from build123d import *
from build123d import SkipClean  # not in build123d's __all__

# Parameters (mm, degrees)
F1_DEPTH = 40
F3_DEPTH = 1.001
F4_DEPTH = 2
F5_DEPTH = 0.5
F6_R     = 0.49999


# Not quite as in the source:
# - a fillet or chamfer is up to 0.001 mm smaller than in the source, because OpenCascade refuses the exact size


with BuildPart() as f1:
    # F0 (on Top) → F1 (new body)
    with BuildSketch(Plane.XY):
        with BuildLine():
            Line((11, 0), (10, 0))
            ThreePointArc((10, 0), (2.4380397486, -9.6982453147), (-8.8111924369, -4.7289415137))
            Line((-8.8111924369, -4.7289415137), (-9.6923116806, -5.2018356651))
            ThreePointArc((-9.6923116806, -5.2018356651), (2.6818437234, -10.6680698462), (11, 0))
        make_face()
        with BuildLine():
            Line((10, 4.582575695), (10, 0))
            Line((10, 0), (11, 0))
            ThreePointArc((11, 0), (10.7470926301, 2.3452078799), (10, 4.582575695))
        make_face()
        with BuildLine():
            Line((10, 16.417424305), (10, 4.582575695))
            ThreePointArc((10, 4.582575695), (10.7470926301, 2.3452078799), (11, 0))
            Line((11, 0), (11, 21))
            ThreePointArc((11, 21), (10.7470926301, 18.6547921201), (10, 16.417424305))
        make_face()
        with BuildLine():
            ThreePointArc((0, 11), (1.6583123952, 10.8742815855), (3.2787192622, 10.5))
            ThreePointArc((3.2787192622, 10.5), (7.2687738933, 12.743794692), (10, 16.417424305))
            Line((10, 16.417424305), (10, 21))
            ThreePointArc((10, 21), (7.0710678119, 13.9289321881), (0, 11))
        make_face()
        with BuildLine():
            ThreePointArc((-3.2787192622, 10.5), (-1.6583124171, 10.1257184179), (-4.44e-08, 10))
            ThreePointArc((-4.44e-08, 10), (1.6583123732, 10.1257184112), (3.2787192622, 10.5))
            ThreePointArc((3.2787192622, 10.5), (1.6583123952, 10.8742815855), (0, 11))
            ThreePointArc((0, 11), (-1.6583123952, 10.8742815855), (-3.2787192622, 10.5))
        make_face()
        with BuildLine():
            ThreePointArc((-9.6923116806, 15.7981643349), (-7.0056796429, 12.5194072884), (-3.2787192622, 10.5))
            ThreePointArc((-3.2787192622, 10.5), (-1.6583123952, 10.8742815855), (0, 11))
            ThreePointArc((0, 11), (-5.1337405886, 12.4183505333), (-8.8111924369, 16.2710584863))
            Line((-8.8111924369, 16.2710584863), (-9.6923116806, 15.7981643349))
        make_face()
        with BuildLine():
            Line((10, 21), (10, 16.417424305))
            ThreePointArc((10, 16.417424305), (10.7470926301, 18.6547921201), (11, 21))
            ThreePointArc((11, 21), (10.7470926301, 23.3452078799), (10, 25.582575695))
            Line((10, 25.582575695), (10, 21))
        make_face()
        with BuildLine():
            ThreePointArc((10, 25.582575695), (10.7470926301, 23.3452078799), (11, 21))
            Line((11, 21), (11, 42))
            ThreePointArc((11, 42), (10.7470926301, 39.6547921201), (10, 37.417424305))
            Line((10, 37.417424305), (10, 25.582575695))
        make_face()
        with BuildLine():
            ThreePointArc((5.81e-08, 32), (1.6583124239, 31.8742815811), (3.2787192622, 31.5))
            ThreePointArc((3.2787192622, 31.5), (7.2687738933, 33.743794692), (10, 37.417424305))
            Line((10, 37.417424305), (10, 42))
            ThreePointArc((10, 42), (7.0710678324, 34.9289322087), (5.81e-08, 32))
        make_face()
        with BuildLine():
            ThreePointArc((5.81e-08, 32), (-1.6583123665, 31.8742815898), (-3.2787192622, 31.5))
            ThreePointArc((-3.2787192622, 31.5), (-1.658312379, 31.1257184121), (3.28e-08, 31))
            ThreePointArc((3.28e-08, 31), (1.6583124114, 31.125718417), (3.2787192622, 31.5))
            ThreePointArc((3.2787192622, 31.5), (1.6583124239, 31.8742815811), (5.81e-08, 32))
        make_face()
        with BuildLine():
            ThreePointArc((-9.6923116806, 36.7981643349), (-7.0056796429, 33.5194072884), (-3.2787192622, 31.5))
            ThreePointArc((-3.2787192622, 31.5), (-1.6583123665, 31.8742815898), (5.81e-08, 32))
            ThreePointArc((5.81e-08, 32), (-5.1337405637, 33.4183505184), (-8.8111924369, 37.2710584863))
            Line((-8.8111924369, 37.2710584863), (-9.6923116806, 36.7981643349))
        make_face()
        with BuildLine():
            ThreePointArc((10, 37.417424305), (10.7470926301, 39.6547921201), (11, 42))
            ThreePointArc((11, 42), (10.7470926301, 44.3452078799), (10, 46.582575695))
            Line((10, 46.582575695), (10, 42))
            Line((10, 42), (10, 37.417424305))
        make_face()
        with BuildLine():
            ThreePointArc((10, 46.582575695), (10.7470926301, 44.3452078799), (11, 42))
            Line((11, 42), (11, 63))
            ThreePointArc((11, 63), (10.7470926301, 60.6547921201), (10, 58.417424305))
            Line((10, 58.417424305), (10, 46.582575695))
        make_face()
        with BuildLine():
            ThreePointArc((10, 58.417424305), (10.7470926301, 60.6547921201), (11, 63))
            ThreePointArc((11, 63), (10.8000300748, 65.0879057409), (10.2073908395, 67.0998990536))
            Line((10.2073908395, 67.0998990536), (10, 67.0998990536))
            Line((10, 67.0998990536), (10, 63))
            Line((10, 63), (10, 58.417424305))
        make_face()
        with BuildLine():
            ThreePointArc((0, 53), (1.6583123952, 52.8742815855), (3.2787192622, 52.5))
            ThreePointArc((3.2787192622, 52.5), (7.2687738933, 54.743794692), (10, 58.417424305))
            Line((10, 58.417424305), (10, 63))
            ThreePointArc((10, 63), (7.0710678119, 55.9289321881), (0, 53))
        make_face()
        with BuildLine():
            ThreePointArc((-5.66e-08, 52), (1.6583123672, 52.1257184103), (3.2787192622, 52.5))
            ThreePointArc((3.2787192622, 52.5), (1.6583123952, 52.8742815855), (0, 53))
            ThreePointArc((0, 53), (-1.6583123952, 52.8742815855), (-3.2787192622, 52.5))
            ThreePointArc((-3.2787192622, 52.5), (-1.6583124232, 52.1257184188), (-5.66e-08, 52))
        make_face()
        with BuildLine():
            ThreePointArc((-9.6923116806, 57.7981643349), (-7.0056796429, 54.5194072884), (-3.2787192622, 52.5))
            ThreePointArc((-3.2787192622, 52.5), (-1.6583123952, 52.8742815855), (0, 53))
            ThreePointArc((0, 53), (-5.1337405886, 54.4183505333), (-8.8111924369, 58.2710584863))
            Line((-8.8111924369, 58.2710584863), (-9.6923116806, 57.7981643349))
        make_face()
        with BuildLine():
            ThreePointArc((10, 67.582575695), (10.1065773297, 67.3424756395), (10.2073908395, 67.0998990536))
            Line((10.2073908395, 67.0998990536), (11, 67.0998990536))
            Line((11, 67.0998990536), (11, 89.784912765))
            Line((11, 89.784912765), (10, 89.784912765))
            Line((10, 89.784912765), (10, 67.582575695))
        make_face()
        with BuildLine():
            ThreePointArc((10.2073908395, 67.0998990536), (10.8000300748, 65.0879057409), (11, 63))
            Line((11, 63), (11, 67.0998990536))
            Line((11, 67.0998990536), (10.2073908395, 67.0998990536))
        make_face()
        with BuildLine():
            Line((10, 67.0998990536), (10.2073908395, 67.0998990536))
            ThreePointArc((10.2073908395, 67.0998990536), (10.1065773297, 67.3424756395), (10, 67.582575695))
            Line((10, 67.582575695), (10, 67.0998990536))
        make_face()
    extrude(amount=F1_DEPTH)

    # F2 (on face) → F3 (cut, through all)
    with BuildSketch(Plane(origin=(10, 0, 0), x_dir=(0, -1, 0), z_dir=(-1, 0, 0))):
        Polygon((-81.784912765, 10.7769520171), (-81.784912765, 0), (-63, 0), align=None)
        with BuildLine():
            Line((-89.784912765, 0), (-81.784912765, 0))
            Line((-81.784912765, 0), (-81.784912765, 10.7769520171))
            Line((-81.784912765, 10.7769520171), (-85.7659138368, 13.0608624119))
            ThreePointArc((-85.7659138368, 13.0608624119), (-88.7076293046, 15.9905117892), (-89.784912765, 20))
            Line((-89.784912765, 20), (-89.784912765, 0))
        make_face()
        with BuildLine():
            Line((-89.784912765, 40), (-89.784912765, 20))
            ThreePointArc((-89.784912765, 20), (-88.7076292465, 24.0094883112), (-85.7659136356, 26.9391377035))
            Line((-85.7659136356, 26.9391377035), (-81.784912765, 29.2230479829))
            Line((-81.784912765, 29.2230479829), (-81.784912765, 40))
            Line((-81.784912765, 40), (-89.784912765, 40))
        make_face()
        Polygon((-81.784912765, 29.2230479829), (-63, 40), (-81.784912765, 40), align=None)
    extrude(amount=-F3_DEPTH, mode=Mode.SUBTRACT)

    # F2 (on face) → F4 (join)
    with BuildSketch(Plane(origin=(10, 0, 0), x_dir=(0, -1, 0), z_dir=(-1, 0, 0))):
        with BuildLine():
            ThreePointArc((-85.7659138368, 13.0608624119), (-83.8448762714, 12.2697638877), (-81.784912765, 12))
            Line((-81.784912765, 12), (-81.784912765, 12.5))
            ThreePointArc((-81.784912765, 12.5), (-89.284912765, 20), (-81.784912765, 27.5))
            Line((-81.784912765, 27.5), (-81.784912765, 28))
            ThreePointArc((-81.784912765, 28), (-83.8448761593, 27.7302361422), (-85.7659136356, 26.9391377035))
            ThreePointArc((-85.7659136356, 26.9391377035), (-88.7076292465, 24.0094883112), (-89.784912765, 20))
            ThreePointArc((-89.784912765, 20), (-88.7076293046, 15.9905117892), (-85.7659138368, 13.0608624119))
        make_face()
        with BuildLine():
            Line((-81.784912765, 12.5), (-81.784912765, 12))
            ThreePointArc((-81.784912765, 12), (-76.1280585155, 14.3431457505), (-73.784912765, 20))
            ThreePointArc((-73.784912765, 20), (-76.1280585155, 25.6568542495), (-81.784912765, 28))
            Line((-81.784912765, 28), (-81.784912765, 27.5))
            ThreePointArc((-81.784912765, 27.5), (-76.4816119061, 25.3033008589), (-74.284912765, 20))
            ThreePointArc((-74.284912765, 20), (-76.4816119061, 14.6966991411), (-81.784912765, 12.5))
        make_face()
    with SkipClean():  # cleaning this boolean's faces spoils the solid; the shape is the same uncleaned
        extrude(amount=F4_DEPTH)

    # F2 (on face) → F5 (cut)
    with BuildSketch(Plane(origin=(10, 0, 0), x_dir=(0, -1, 0), z_dir=(-1, 0, 0))):
        with BuildLine():
            Line((-81.784912765, 27.5), (-81.784912765, 12.5))
            ThreePointArc((-81.784912765, 12.5), (-76.4816119061, 14.6966991411), (-74.284912765, 20))
            ThreePointArc((-74.284912765, 20), (-76.4816119061, 25.3033008589), (-81.784912765, 27.5))
        make_face()
        with BuildLine():
            ThreePointArc((-81.784912765, 27.5), (-89.284912765, 20), (-81.784912765, 12.5))
            Line((-81.784912765, 12.5), (-81.784912765, 27.5))
        make_face()
    with SkipClean():  # cleaning this boolean's faces spoils the solid; the shape is the same uncleaned
        extrude(amount=-F5_DEPTH, mode=Mode.SUBTRACT)

    # F6 (radius 0.5 in the source; OpenCascade refuses exactly that, so slightly less here)
    f6_edges = [f1.edges().sort_by_distance(p)[0] for p in [
        (-8.811192, 58.271058, 20),
        (-9.692312, 57.798164, 20),
        (-8.811192, 37.271058, 20),
        (-9.692312, 36.798164, 20),
        (-8.811192, 16.271058, 20),
        (-9.692312, 15.798164, 20),
        (-8.811192, -4.728942, 20),
        (-9.692312, -5.201836, 20),
    ]]
    fillet(f6_edges, radius=F6_R)


solid = f1.part
The model under review builds one solid part; all positions refer to its coordinate system, in mm. A direction names the side the tool comes from. Round coordinates to 2 decimals unless told otherwise and drop trailing zeros. Write each loop counter-clockwise with the first axis right and the second up, starting at its lowest first coordinate (ties: lowest second). Pieces come first, ordered by that corner, then holes. Notation, with made-up numbers: (47, -32.5) -> (67, -32.5) arc R22 ccw to (67, -5.5) -> close; hole circle Ø9 at (0.5, 76). An arc over 180 degrees is marked (long way). Answer as a JSON object with one key per item and string values.
1. We need section D-D on x = 4.5. State the section outline as (y, z) points.
Results found:
{"outline": "(-10.04, 0) -> (-8.93, 0) -> (-8.93, 40) -> (-10.04, 40) -> close; (10.96, 0) -> (12.07, 0) -> (12.07, 40) -> (10.96, 40) -> close; (31.96, 0) -> (33.07, 0) -> (33.07, 40) -> (31.96, 40) -> close; (52.96, 0) -> (54.07, 0) -> (54.07, 40) -> (52.96, 40) -> close"}
2. We need section C-C on y = 50. State the section outline as (x, z) points.
Results found:
{"outline": "(10, 0) -> (11, 0) -> (11, 40) -> (10, 40) -> close"}
3. Machinability: for faces 5 (the face through (8, 77, 14)), 6 (the face through (10, 50, 20)), 7 (the face through (3, 32, 40)), which of the approach directions +Z, -Z, +X, -X, +Y, -Y give a long, thin tool a straight path to every point of the face, cutting with its end or side? Answer none if there is none.
Results found:
{"face 5": "+Z, -Z, -X, +Y", "face 6": "+Z, -Z", "face 7": "+Z, +X, -X, +Y, -Y"}
4. We need section B-B on y = 13. State the section outline as (x, z) points.
Results found:
{"outline": "(-7.55, 0) -> (-6, 0) -> (-6, 40) -> (-7.55, 40) -> close; (6, 0) -> (7.55, 0) -> (7.55, 40) -> (6, 40) -> close; (10, 0) -> (11, 0) -> (11, 40) -> (10, 40) -> close"}
5. Clearance check with flat-ended pins moving along their axes: pin 1 (17 mm diameter, centred on y = 81.78, z = 20, fed in from -X); pin 2 (1.5 mm diameter, centred on x = 1.5, z = 12.5, fed in from -Y); pin 3 (13 mm diameter, centred on y = 5.5, z = 17.5, fed in from -X). State where each tip first meets the part, or that it passes through.
Results found:
{"pin 1": "stops at x = 8", "pin 2": "stops at y = -10.97", "pin 3": "stops at x = -6.32"}
6. The part is to be moulded in two halves that separate along X. For faces 1 (the face through (10, 8, 20)), 2 (the face through (10.5, 82, 20)), 3 (the face through (10, 29, 20)), 4 (the face through (11, 44, 20)), say which applies: pulls with the +X half, pulls with the -X half, needs draft (parallel to the pull), parting line crosses it, or undercut.
Results found:
{"face 1": "undercut", "face 2": "pulls with the -X half", "face 3": "undercut", "face 4": "pulls with the +X half"}
7. To check wall thickness, follow line 1 along Y through (x, z) = (9.2, 20); line 2 along X through (y, z) = (57, 11.5); line 3 along Y through (x, z) = (8.85, 20). State the ranges of each line that lie inside material, in increasing order.
Results found:
{"line 1": "y = -6.03 to -3.92, 14.97 to 17.08, 35.97 to 38.08, 56.97 to 59.08, 73.78 to 74.28, 89.28 to 89.78", "line 2": "x = -9.22 to -8, 8 to 9.22, 10 to 11", "line 3": "y = -6.53 to -4.66, 14.47 to 16.34, 35.47 to 37.34, 56.47 to 58.34, 73.78 to 74.28, 89.28 to 89.78"}
8. We need section A-A on x = -1.5. State the section outline as (y, z) points.
Results found:
{"outline": "(-10.9, 0) -> (-9.89, 0) -> (-9.89, 40) -> (-10.9, 40) -> close; (10.1, 0) -> (11.11, 0) -> (11.11, 40) -> (10.1, 40) -> close; (31.1, 0) -> (32.11, 0) -> (32.11, 40) -> (31.1, 40) -> close; (52.1, 0) -> (53.11, 0) -> (53.11, 40) -> (52.1, 40) -> close"}
